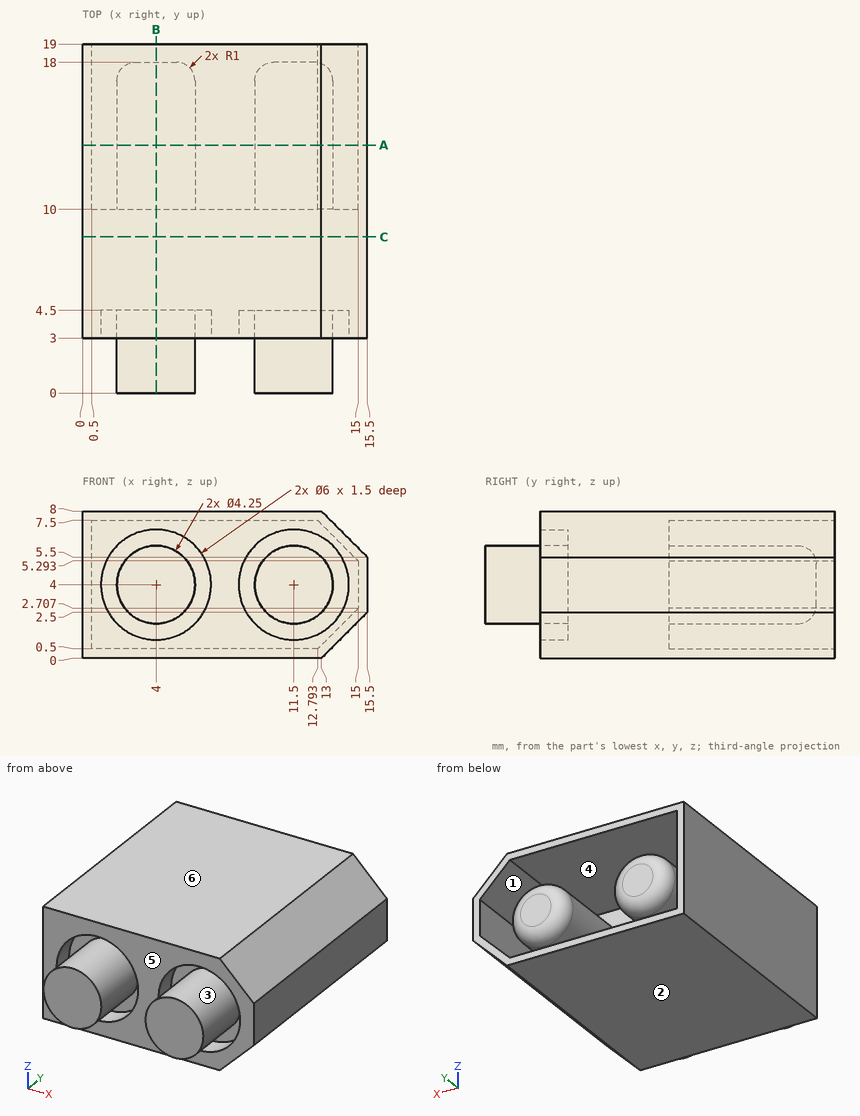
Drawing for the job (mm, zero at the part's lowest x, y, z). A direction names the side the tool comes from. Coordinates: 2 decimals unless noted, no trailing zeros. Loops run counter-clockwise (first coordinate to the right, second up) from the corner with the lowest first, then second, coordinate; pieces in that order, holes last. Notation, with made-up numbers: (27.25, 65) - (55.25, 65) arc R20 cw to (55.25, 89) - close; hole circle Ø5 at (-18.5, 9). An arc over 180 degrees is marked (long way). Return JSON: item names as keys, results as strings.
1. Band-saw the part on A-A (y = 13.5). Give the cut face in (x, z) (3 decimals), and give its area (3 significant figures).
Result:
{"outline": "(0, 0) - (13, 0) - (15.5, 2.5) - (15.5, 5.5) - (13, 8) - (0, 8) - close; circle Ø4.25 at (4, 4); circle Ø4.25 at (11.5, 4); hole (0.5, 0.5) - (12.793, 0.5) - (15, 2.707) - (15, 5.293) - (12.793, 7.5) - (0.5, 7.5) - close", "area": "49.5 mm2"}
2. Band-saw the part on B-B (x = 4). Give the cut face in (y, z) (3 decimals), and give its area (3 significant figures).
Result:
{"outline": "(0, 1.875) - (4.5, 1.875) - (4.5, 1) - (3, 1) - (3, 0) - (19, 0) - (19, 0.5) - (10, 0.5) - (10, 1.875) - (17, 1.875) arc R1 ccw to (18, 2.875) - (18, 5.125) arc R1 ccw to (17, 6.125) - (10, 6.125) - (10, 7.5) - (19, 7.5) - (19, 8) - (3, 8) - (3, 7) - (4.5, 7) - (4.5, 6.125) - (0, 6.125) - close", "area": "109 mm2"}
3. Drop flat-ended pins along their axis: pin 1 (1.8 mm diameter, centred on x = 4.5, z = 4, fed in from +Y); pin 2 (1.5 mm diameter, centred on y = 10.5, z = 6.5, fed in from +X). Give the stop position or say it passes through.
Result:
{"pin 1": "stops at y = 18", "pin 2": "stops at x = 15.25"}
4. Probe L1, parallel to X at y = 3.9, z = 4 (3 decimals); L2, parallel to Z at x = 11.5, y = 4.2 (3 decimals); L3, parallel to Y at x = 7.5, z = 3.75. List the from-to ranges inside material, lowest first. Write a range as from..to.
Result:
{"L1": "x = 0..1, 1.875..6.125, 7..8.5, 9.375..13.625, 14.5..15.5", "L2": "z = 0..1, 1.875..6.125, 7..8", "L3": "y = 3..10"}
5. 3-axis set-ups, long thin cutter, end or side, ignore diameter. For the marked faces 1, 2 and 3: which of +Z, -Z, +X, -X, +Y, -Y reach the whole face in a straight line?
Result:
{"face 1": "+Y", "face 2": "-Z, +X, -X, +Y, -Y", "face 3": "-Y"}
6. Band-saw the part on C-C (y = 8.5). Give the cut face in (x, z), and give its area (3 significant figures).
Result:
{"outline": "(0, 0) - (13, 0) - (15.5, 2.5) - (15.5, 5.5) - (13, 8) - (0, 8) - close", "area": "118 mm2"}
7. Mould opens along Z. For the marked faces 4, 5 and 6 say: released by +Z, released by -Z, zero draft, split by the parting line, or undercut.
Result:
{"face 4": "undercut", "face 5": "zero draft", "face 6": "released by +Z"}
